from build123d import *

# Parameters (mm, degrees)
SKETCH1_R           = 1.5
SKETCH1_R_2         = 10.5
BOSS_EXTRUDE1_DEPTH = 5
SKETCH1_3_R         = 10.5
SKETCH1_3_R_2       = 9.5
BOSS_EXTRUDE2_DEPTH = 4
SKETCH3_3_R         = 9.5
CUT_EXTRUDE2_DEPTH  = 5
SKETCH3_R           = 10.5
SKETCH3_R_2         = 9.5
CUT_EXTRUDE3_DEPTH  = 1


with BuildPart() as part:
    # Sketch1 → Boss-Extrude1 (new body)
    # profile 1 of 2: a face of its own
    with BuildSketch(Plane.XY):
        Polygon((-25, 0), (0, 0), (50, 0), (60, 0), (60, 140), (50, 140), (50, 75), (-25, 75), align=None)
        with Locations((-21.5, 9)):
            Circle(SKETCH1_R, mode=Mode.SUBTRACT)
        with Locations((-12.5, 62.5)):
            Circle(SKETCH1_R_2, mode=Mode.SUBTRACT)
        with Locations((56.5, 9)):
            Circle(SKETCH1_R, mode=Mode.SUBTRACT)
        with Locations((56.5, 134)):
            Circle(SKETCH1_R, mode=Mode.SUBTRACT)
    # profile 2 of 2: a face of its own
    with BuildSketch(Plane.XY):
        Polygon((25, 140), (-25, 75), (50, 75), (50, 140), align=None)
    extrude(amount=BOSS_EXTRUDE1_DEPTH)

    # Sketch1<3> → Boss-Extrude2 (add)
    with BuildSketch(Plane.XY):
        with Locations((-12.5, 62.5)):
            Circle(SKETCH1_3_R)
        with Locations((-12.5, 62.5)):
            Circle(SKETCH1_3_R_2, mode=Mode.SUBTRACT)
    extrude(amount=BOSS_EXTRUDE2_DEPTH)

    # Sketch3<3> → Cut-Extrude2 (cut)
    with BuildSketch(Plane.XY.offset(5)):
        with Locations((30, 30)):
            Circle(SKETCH3_3_R)
    extrude(amount=-CUT_EXTRUDE2_DEPTH, mode=Mode.SUBTRACT)

    # Sketch3 → Cut-Extrude3 (cut)
    with BuildSketch(Plane.XY.offset(5)):
        with Locations((30, 30)):
            Circle(SKETCH3_R)
        with Locations((30, 30)):
            Circle(SKETCH3_R_2, mode=Mode.SUBTRACT)
    extrude(amount=-CUT_EXTRUDE3_DEPTH, mode=Mode.SUBTRACT)


solid = part.part
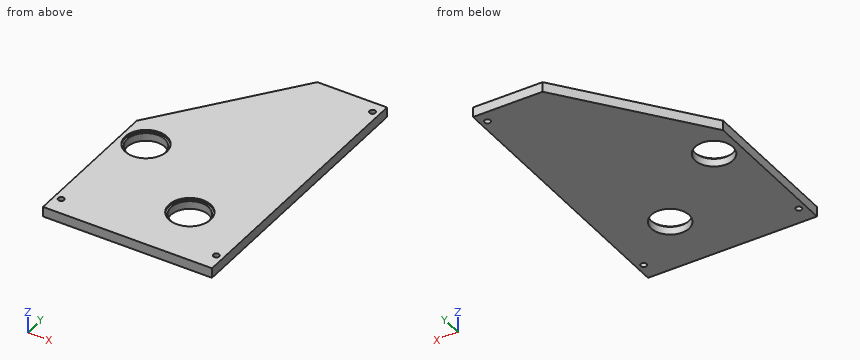
For this review, take the finished solid that the model builds, in its own axes (mm). Give positions to 0.01 mm unless a question says otherwise; leave off trailing zeros. Loops run counter-clockwise (first coordinate to the right, second up) from the corner with the lowest first, then second, coordinate; pieces in that order, holes last.
Item 1: For line 1 along Y through (x, z) = (56.5, 3.7); line 2 along Y through (x, z) = (30, 4.5); line 3 along X through (y, z) = (134, 2.2), list the stretches that pass through material, from the lowest coordinate up.
Item 2: Take a section at A-A, the plane y = 9. State the section outline as (x, z) points.
Item 3: Insertion check: pin 1 (1.5 mm diameter, centred on y = 94, z = 4, fed in from -X); pin 2 (1.5 mm diameter, centred on x = -9.5, z = 3.5, fed in from +Y) (3 decimals); pin 3 (6.5 mm diameter, centred on x = -10.5, y = 65.5, fed in from +Z). Each pin has a flat end and moves straight along its axis. Give the tip position at first contact, or say it passes through.
Item 4: Take a section at C-C, the plane x = -13. State the section outline as (y, z) points.
Item 5: Take a section at B-B, the plane z = 0.8. State the section outline as (x, y) points.
Item 6: Take a section at D-D, the plane y = 30. State the section outline as (x, z) points.
Calculated:
1. line 1: y = 0 to 7.5, 10.5 to 132.5, 135.5 to 140
1. line 2: y = 0 to 19.5, 40.5 to 140
1. line 3: x = 20.38 to 55, 58 to 60
2. outline: (-25, 0) - (-23, 0) - (-23, 5) - (-25, 5) - close; (-20, 0) - (55, 0) - (55, 5) - (-20, 5) - close; (58, 0) - (60, 0) - (60, 5) - (58, 5) - close
3. pin 1: stops at x = -10.96
3. pin 2: stops at y = 96.125
3. pin 3: passes through
4. outline: (0, 0) - (53.01, 0) - (53.01, 4) - (52.01, 4) - (52.01, 5) - (0, 5) - close; (71.99, 0) - (90.6, 0) - (90.6, 5) - (72.99, 5) - (72.99, 4) - (71.99, 4) - close
5. outline: (-25, 0) - (60, 0) - (60, 140) - (25, 140) - (-25, 75) - close; hole circle Ø3 at (-21.5, 9); hole circle Ø19 at (-12.5, 62.5); hole circle Ø19 at (30, 30); hole circle Ø3 at (56.5, 9); hole circle Ø3 at (56.5, 134)
6. outline: (-25, 0) - (20.5, 0) - (20.5, 4) - (19.5, 4) - (19.5, 5) - (-25, 5) - close; (39.5, 0) - (60, 0) - (60, 5) - (40.5, 5) - (40.5, 4) - (39.5, 4) - close
